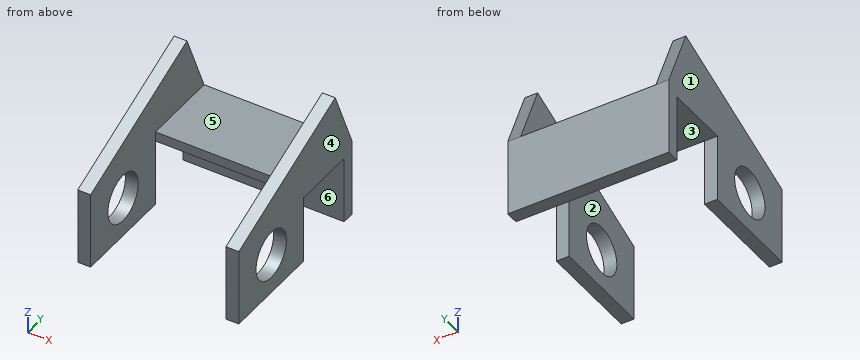
```python
from build123d import *

# Parameters (mm, degrees)
F0_W     = 63.5
F0_H     = 30.48
F1_DEPTH = 71.12
F2_W     = 53.34
F2_H     = 30.48
F3_DEPTH = 40.64
F4_R     = 9.525
F4_W     = 25.4
F4_H     = 26.6478173435
F5_DEPTH = 63.5
F7_DEPTH = 5.08
F9_DEPTH = 5.08


# Not quite as in the source:
# - a feature names something its author has since deleted; it is built from what else it names


with BuildPart() as f1:
    # F0 (on Front) → F1 (new body)
    with BuildSketch(Plane.XZ):
        with Locations((31.75, 15.24)):
            Rectangle(F0_W, F0_H)
    extrude(amount=F1_DEPTH)

    # F2 (on face) → F3 (cut)
    with BuildSketch(Plane.XZ.offset(71.12)):
        with Locations((31.75, 15.24)):
            Rectangle(F2_W, F2_H)
    extrude(amount=-F3_DEPTH, mode=Mode.SUBTRACT)

    # F4 (on face) → F5 (cut)
    with BuildSketch(Plane.YZ.offset(63.5)):
        with Locations((-50.8, 15.8844571561)):
            Circle(F4_R)
        with Locations((-17.78, 13.3239086717)):
            Rectangle(F4_W, F4_H)
    extrude(amount=-F5_DEPTH, mode=Mode.SUBTRACT)

    # F6 (on face) → F7 (join)
    with BuildSketch(Plane.YZ.offset(63.5)):
        Polygon((-10.6731842133, 55.88), (-71.12, 30.48), (0, 30.48), align=None)
    extrude(amount=-F7_DEPTH)

    # F8 (on face) → F9 (join)
    with BuildSketch(Plane(origin=(0, 0, 0), x_dir=(0, -1, 0), z_dir=(-1, 0, 0))):
        Polygon((10.6731842133, 55.88), (0, 30.48), (71.12, 30.48), align=None)
    extrude(amount=-F9_DEPTH)


solid = f1.part
```
The model under review builds one solid part; all positions refer to its coordinate system, in mm. Face numbers are marked on the shaded views. A direction names the side the tool comes from. Round coordinates to 2 decimals unless told otherwise and drop trailing zeros. Order: outer loops, then holes, each group sorted by start corner. A loop starts at its lowest first (then second) coordinate and runs counter-clockwise, first axis right, second up.
Item 1: Machinability: for the marked faces 1, 2 and 3, which of the approach directions +Z, -Z, +X, -X, +Y, -Y give a long, thin tool a straight path to every point of the face, cutting with its end or side? Answer none if there is none.
Working result:
face 1: +Z, -Z, -X, +Y, -Y
face 2: +Z, -Y
face 3: -Z, +X, -X
Item 2: For pin 1 (2 mm diameter, centred on y = -38.5, z = 26.5, fed in from -X); pin 2 (2 mm diameter, centred on x = 10.5, y = -32.5, fed in from +Z); pin 3 (8 mm diameter, centred on x = 46.5, z = 12, fed in from -Y); pin 4 (7.5 mm diameter, centred on x = 16.5, y = -20, fed in from -Z), all flat-tipped, find the tip position at first contact; note any pin that passes through.
Working result:
pin 1: stops at x = 0
pin 2: passes through
pin 3: stops at y = -5.08
pin 4: stops at z = 26.65
Item 3: To check wall thickness, follow probe 1 along X at (y, z) = (-63.5, 33.5); probe 2 along Y at (x, z) = (46.5, 12.5); probe 3 along Y at (x, z) = (34.5, 29.5). State the ranges of each line that lie inside material, in increasing order.
Working result:
probe 1: x = 0 to 5.08, 58.42 to 63.5
probe 2: y = -5.08 to 0
probe 3: y = -30.48 to 0
Item 4: Draft analysis for pull direction X (two halves, no side actions). For the marked faces 4, 5 and 6, state which applies: released by +X, released by -X, zero draft, split by the parting line, or undercut.
Working result:
face 4: released by +X
face 5: undercut
face 6: zero draft
Item 5: Add section B-B, the plane y = -37. State the section outline as (x, z) points, and give its area (3 significant figures).
Working result:
outline: (0, 0) - (5.08, 0) - (5.08, 44.82) - (0, 44.82) - close; (58.42, 0) - (63.5, 0) - (63.5, 44.82) - (58.42, 44.82) - close
area: 455 mm2
Item 6: Add section D-D, the plane y = -50.8. State the section outline as (x, z) points, and give its area (3 significant figures).
Working result:
outline: (0, 0) - (5.08, 0) - (5.08, 6.36) - (0, 6.36) - close; (0, 25.41) - (5.08, 25.41) - (5.08, 39.02) - (0, 39.02) - close; (58.42, 0) - (63.5, 0) - (63.5, 6.36) - (58.42, 6.36) - close; (58.42, 25.41) - (63.5, 25.41) - (63.5, 39.02) - (58.42, 39.02) - close
area: 203 mm2
Item 7: Add section C-C, the plane z = 42. State the section outline as (x, y) points, and give its area (3 significant figures).
Working result:
outline: (0, -43.7) - (5.08, -43.7) - (5.08, -4.84) - (0, -4.84) - close; (58.42, -43.7) - (63.5, -43.7) - (63.5, -4.84) - (58.42, -4.84) - close
area: 395 mm2
Item 8: Add section A-A, the plane z = 8.5. State the section outline as (x, y) points.
Working result:
outline: (0, -71.12) - (5.08, -71.12) - (5.08, -56.82) - (0, -56.82) - close; (0, -44.78) - (5.08, -44.78) - (5.08, -30.48) - (0, -30.48) - close; (0, -5.08) - (63.5, -5.08) - (63.5, 0) - (0, 0) - close; (58.42, -71.12) - (63.5, -71.12) - (63.5, -56.82) - (58.42, -56.82) - close; (58.42, -44.78) - (63.5, -44.78) - (63.5, -30.48) - (58.42, -30.48) - close
